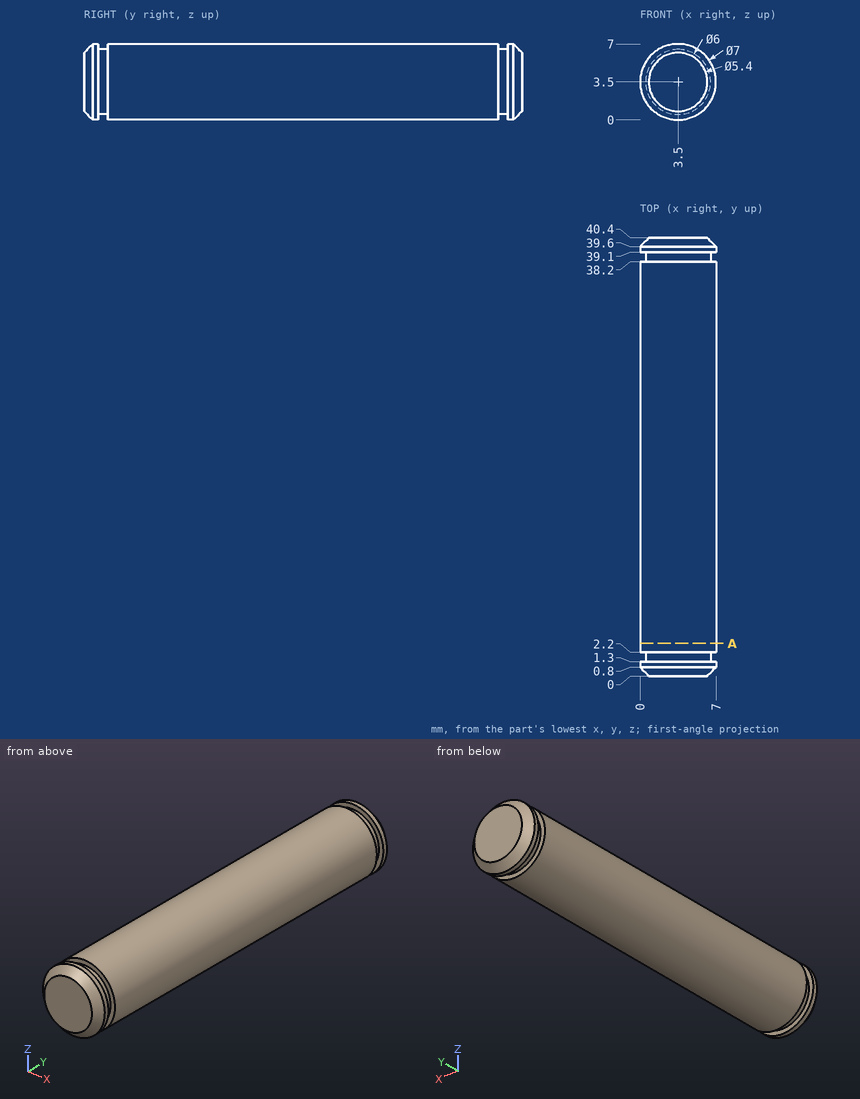
Answer from the drawing. Dimensions are ordinates in mm from the lowest x, y and z of the part. Coordinates: 2 decimals unless noted, no trailing zeros. Loops run counter-clockwise (first coordinate to the right, second up) from the corner with the lowest first, then second, coordinate; pieces in that order, holes last.
1) Section A-A (y = 3) is taken. Give the vertices of the cut face in (x, z), plus the area to 3 significant figures.
Results:
outline: circle Ø7 at (3.5, 3.5)
area: 38.5 mm2
2) Flat-ended cylindrical pins translate along their axes: pin 1 (1.5 mm diameter, centred on x = 6, y = 7, fed in from +Z); pin 2 (1 mm diameter, centred on x = 2, y = 4, fed in from +Z); pin 3 (2 mm diameter, centred on x = 1.5, y = 23, fed in from -Z). Find the tip coordinate at first contact, or state that the pin passes through.
Results:
pin 1: stops at z = 6.53
pin 2: stops at z = 6.85
pin 3: stops at z = 0.15
3) Consider probe 1 along Y at (x, z) = (1.5, 6); probe 2 along Y at (x, z) = (6, 1.25); probe 3 along Z at (x, y) = (3.75, 21). Determine where each line is inside the solid, lowest interval first.
Results:
probe 1: y = 0.5 to 1.3, 2.2 to 38.2, 39.1 to 39.9
probe 2: y = 0.66 to 1.3, 2.2 to 38.2, 39.1 to 39.74
probe 3: z = 0.01 to 6.99
